from build123d import *

# Parameters (mm, degrees)
SKETCH_1_W                     = 145
SKETCH_1_H                     = 80
EXTRUDE_1_DEPTH                = 3
SKETCH_3_R                     = 3
EXTRUDE_2_DEPTH                = 2
HOLE_WIZARD_M3_5_4_D           = 2.9
HOLE_WIZARD_M3_5_4_DEPTH       = 11.2
HOLE_WIZARD_M3_5_4_CSINK_D     = 3.55
HOLE_WIZARD_M3_5_4_CSINK_ANGLE = 90
HOLE_WIZARD_M3_5_4_TIP         = 0.871247898
HOLE_WIZARD_M3_5_5_D           = 2.9
HOLE_WIZARD_M3_5_5_DEPTH       = 7
HOLE_WIZARD_M3_5_5_CSINK_D     = 3.55
HOLE_WIZARD_M3_5_5_CSINK_ANGLE = 90
HOLE_WIZARD_M3_5_5_TIP         = 0.871247898
HOLE_WIZARD_M3_5_7_D           = 2.9
HOLE_WIZARD_M3_5_7_CSINK_D     = 3.55
HOLE_WIZARD_M3_5_7_CSINK_ANGLE = 90


with BuildPart() as part:
    # 草图1 → 凸台-拉伸1 (new body)
    with BuildSketch(Plane(origin=(0, 0, 0), x_dir=(1, 0, 0), z_dir=(0, 1, 0))):
        with Locations((72.5, 40)):
            Rectangle(SKETCH_1_W, SKETCH_1_H)
    extrude(amount=EXTRUDE_1_DEPTH)

    # 草图3 → 凸台-拉伸2 (add)
    with BuildSketch(Plane(origin=(0, 3, 0), x_dir=(1, 0, 0), z_dir=(0, 1, 0))):
        with Locations(Location((59.085, 63.5, 0), (0, 0, 90))):
            Circle(SKETCH_3_R)
        with Locations(Location((59.085, 16.5, 0), (0, 0, 90))):
            Circle(SKETCH_3_R)
        with Locations(Location((141.915, 16.5, 0), (0, 0, 90))):
            Circle(SKETCH_3_R)
        with Locations(Location((141.915, 63.5, 0), (0, 0, 90))):
            Circle(SKETCH_3_R)
        with Locations(Location((6, 62, 0), (0, 0, 90))):
            Circle(SKETCH_3_R)
        with Locations(Location((50, 62, 0), (0, 0, 90))):
            Circle(SKETCH_3_R)
        with Locations(Location((6, 18, 0), (0, 0, 90))):
            Circle(SKETCH_3_R)
        with Locations(Location((50, 18, 0), (0, 0, 90))):
            Circle(SKETCH_3_R)
    extrude(amount=EXTRUDE_2_DEPTH)

    # M3.5 螺纹孔4
    with Locations(Plane(origin=(0, 5, 0), x_dir=(1, 0, 0), z_dir=(0, 1, 0))):
        with Locations((141.915, 63.5), (6, 62), (50, 62), (59.085, 63.5), (50, 18), (6, 18), (141.915, 16.5), (59.085, 16.5)):
            CounterSinkHole(HOLE_WIZARD_M3_5_4_D / 2, HOLE_WIZARD_M3_5_4_CSINK_D / 2, depth=HOLE_WIZARD_M3_5_4_DEPTH, counter_sink_angle=HOLE_WIZARD_M3_5_4_CSINK_ANGLE)
            with Locations((0, 0, -(HOLE_WIZARD_M3_5_4_DEPTH + HOLE_WIZARD_M3_5_4_TIP / 2))):  # 118° drill point
                Cone(0, HOLE_WIZARD_M3_5_4_D / 2, HOLE_WIZARD_M3_5_4_TIP, mode=Mode.SUBTRACT)

    # M3.5 螺纹孔5
    with Locations(Plane.XZ):
        with Locations((86.5, -56), (38, -5), (30, -70), (115, -70), (115, -10), (30, -10), (56.5, -56)):
            CounterSinkHole(HOLE_WIZARD_M3_5_5_D / 2, HOLE_WIZARD_M3_5_5_CSINK_D / 2, depth=HOLE_WIZARD_M3_5_5_DEPTH, counter_sink_angle=HOLE_WIZARD_M3_5_5_CSINK_ANGLE)
            with Locations((0, 0, -(HOLE_WIZARD_M3_5_5_DEPTH + HOLE_WIZARD_M3_5_5_TIP / 2))):  # 118° drill point
                Cone(0, HOLE_WIZARD_M3_5_5_D / 2, HOLE_WIZARD_M3_5_5_TIP, mode=Mode.SUBTRACT)

    # M3.5 螺纹孔7 (through all)
    with Locations(Plane(origin=(0, 3, 0), x_dir=(1, 0, 0), z_dir=(0, 1, 0))):
        with Locations((5, 75), (140, 75), (140, 5), (5, 5)):
            CounterSinkHole(HOLE_WIZARD_M3_5_7_D / 2, HOLE_WIZARD_M3_5_7_CSINK_D / 2, counter_sink_angle=HOLE_WIZARD_M3_5_7_CSINK_ANGLE)


solid = part.part
The listing builds one solid part. Answer for the finished solid, in the listing's coordinates (mm). Give positions to 0.01 mm unless a question says otherwise; leave off trailing zeros. Write each loop counter-clockwise with the first axis right and the second up, starting at its lowest first coordinate (ties: lowest second). Pieces come first, ordered by that corner, then holes.
Item 1: Determine the mould class of faces 1 (the flat face through (71, 1, -80)), 2 (the cylindrical face through (140.576, 2.305, -15.945)), 3 (the cylindrical face through (39.45, 1.68, -4.94)) for opening direction X: released by +X, released by -X, zero draft, split by the parting line, or undercut.
Item 2: Section A-A, the plane x = 38 is taken. Write down the section's boundary in (y, z) (3 decimals), plus the area to 3 significant figures.
Item 3: Section B-B, the plane z = -52 is taken. Write down the section's boundary in (x, y), plus the area to 3 significant figures.
Item 4: Section C-C, the plane x = 104 is taken. Write down the section's boundary in (y, z).
Item 5: Flat-ended cylindrical pins translate along their axes: P1, Ø3.5, axis at x = 30, z = -70, coming from the -Y side (3 decimals); P2, Ø8, axis at x = 20.5, z = -38.5, coming from the +Y side; P3, Ø2, axis at y = 4.5, z = -62, coming from the +X side. Find the tip coordinate at first contact, or state that the pin passes through.
Item 6: Find the intervals of material crossed by line 1 along X through (y, z) = (1.1, -5); line 2 along X through (y, z) = (1.9, -70); line 3 along Z through (x, y) = (140, 1.3), in increasing order.
Completed:
1. face 1: zero draft
1. face 2: undercut
1. face 3: undercut
2. outline: (0, -80) - (3, -80) - (3, -6.45) - (0.325, -6.45) - (0, -6.775) - close; (0, -3.225) - (0.325, -3.55) - (3, -3.55) - (3, 0) - (0, 0) - close
2. area: 231 mm2
3. outline: (0, 0) - (145, 0) - (145, 3) - (0, 3) - close
3. area: 435 mm2
4. outline: (0, -80) - (3, -80) - (3, 0) - (0, 0) - close
5. P1: stops at y = 0.025
5. P2: stops at y = 3
5. P3: stops at x = 144.87
6. line 1: x = 0 to 3.55, 6.45 to 36.55, 39.45 to 138.55, 141.45 to 145
6. line 2: x = 0 to 28.55, 31.45 to 113.55, 116.45 to 145
6. line 3: z = -80 to -76.45, -73.55 to -6.45, -3.55 to 0
